Can you work these out from the model? Positions are in its coordinate system, mm. Round coordinates to 2 decimals unless told otherwise and drop trailing zeros. Loops run counter-clockwise (first coordinate to the right, second up) from the corner with the lowest first, then second, coordinate; pieces in that order, holes last.
(1) If I drill on line 1 along Z through (x, y) = (-2009, -2.5); line 2 along Z through (x, y) = (-1565, -0.5); line 3 along X through (y, z) = (63, 90), over which ranges is the centre line in solid material (lowest first)?
(2) Will these pins go through, and if not, where does the flat tip stop? pin 1 Ø3 at (x, y) = (-1122.5, 13) entering from +Z; pin 2 Ø2 at (x, z) = (-1556.5, 10) entering from -Y; pin 3 Ø1.5 at (x, z) = (-1864.5, 6) entering from +Y.
(3) I want a section at A-A on x = -290.5. Write out the boundary of the cut face in (y, z), plus the area to 3 significant figures.
from build123d import *

# Parameters (mm, degrees)
CROQUIS1_R = 13.7


with BuildPart() as part:
    # Barrer1: sweep along a curve in space
    with BuildLine() as barrer1_path:
        Line((0, 0, 0), (-2374, 0, 0))
        ThreePointArc((-2374, 0, 0), (-2384.606601718, 4.393398282, 0), (-2389, 15, 0))
        Line((-2389, 15, 0), (-2389, 25, 0))
        ThreePointArc((-2389, 25, 0), (-2389, 35.606601718, 4.393398282), (-2389, 40, 15))
        Line((-2389, 40, 15), (-2389, 40, 82.5))
        ThreePointArc((-2389, 40, 82.5), (-2389, 44.393398282, 93.106601718), (-2389, 55, 97.5))
        Line((-2389, 55, 97.5), (-2389, 90, 97.5))
    # Croquis1 → Barrer1 (sweep)
    with BuildSketch(Plane(origin=(0, 0, 0), x_dir=(0, 0, -1), z_dir=(1, 0, 0))):
        Circle(CROQUIS1_R)
    sweep(path=barrer1_path.line)


solid = part.part
Filled sheet:
1. line 1: z = -13.47 to 13.47
1. line 2: z = -13.69 to 13.69
1. line 3: x = -2400.46 to -2377.54
2. pin 1: stops at z = 7.45
2. pin 2: stops at y = -10.33
2. pin 3: stops at y = 12.65
3. outline: circle Ø27.4 at (0, 0)
3. area: 590 mm2
